Autodesk Inventor part; units mm, degrees
ref_plane "YZ Plane" through (0, 0, 0) normal (1, 0, 0) x (0, 1, 0)
ref_plane "XZ Plane" through (0, 0, 0) normal (0, 1, 0) x (-1, 0, 0)
ref_plane "XY Plane" through (0, 0, 0) normal (0, 0, 1) x (1, 0, 0)
sketch "Sketch1" plane through (0, 0, 0) normal (0, 0, 1) x (1, 0, 0)
  line L0 (0, 0) -> (18, 0)
  line L1 (18, 0) -> (18, 24)
  line L2 (18, 24) -> (0, 24)
  line L3 (0, 24) -> (0, 0)
  circle A0 centre (15, 21) radius 1.05
  circle A1 centre (5, 2.5) radius 1.05
  circle A2 centre (3, 7) radius 1.05
  line L4 (0, 10) -> (11.3137, 10) construction
  line L5 (6, 0) -> (28.3492, 0) construction
  line L6 (6, 0) -> (42, 0) construction
  circle A3 centre (9.749, 12) radius 1
  circle A4 centre (15, 21) radius 2.75
  circle A5 centre (5, 5) radius 5
  line L7 (1.1063, 8.1367) -> (12.8585, 22.7252)
  circle A6 centre (5, 2.5) radius 2.5
  line L8 (7.185, 1.2851) -> (17.4035, 19.6637)
  point P0 (8, 24)
  point P1 (18, 31.1769)
  point P2 (9.5257, 2.8745)
  point P3 (17.4892, 19.831)
  point P4 (5, 0)
  dimension "d0" = 18
  dimension "d1" = 24
  dimension "d2" = 2.1
  dimension "d3" = 3
  dimension "d4" = 3
  dimension "d5" = 2.1
  dimension "d6" = 2.1
  dimension "d7" = 2.5
  dimension "d8" = 5
  dimension "d9" = 3
  dimension "d10" = 7
  dimension "d12" = 10
  dimension "d15" = 6
  dimension "d18" = 2
  dimension "d25" = 5.5
  dimension "d26" = 10
  dimension "d30" = 12
  dimension "d31" = 8.251
extrude "Extrusion1" add sketch "Sketch1" along normal blind 8 contours A5 L8 A6 | A6 | L7 A4 L8 A5 | A4 picked at (5.8937, 6.9979)
sketch "Sketch3" plane through (0, 0, 0) normal (0, 0, -1) x (-1, 0, 0)
  circle A0 centre (-9.749, 12) radius 1
  circle A1 centre (-9.749, 12) radius 7.45
  point P0 (0, 0)
  dimension "d27" = 14.9
extrude "Extrusion2" cut sketch "Sketch3" against normal blind 2.7
sketch "Sketch5" plane through (0, 0, 8) normal (0, 0, 1) x (1, 0, 0)
  circle A0 centre (3, 7) radius 1.05
  circle A1 centre (5, 2.5) radius 1.05
  circle A2 centre (15, 21) radius 1.05
  circle A3 centre (3, 7) radius 2
  circle A4 centre (5, 2.5) radius 2
  circle A5 centre (15, 21) radius 2
  point P0 (0, 0)
  dimension "d32" = 4
  dimension "d33" = 4
  dimension "d34" = 4
extrude "Extrusion3" cut sketch "Sketch5" against normal blind 4.9
sketch "Sketch6" plane through (0, 0, 2.7) normal (0, 0, -1) x (-1, 0, 0)
  circle A0 centre (-9.749, 12) radius 1
  circle A1 centre (-9.749, 12) radius 1
  circle A2 centre (-9.749, 12) radius 5.7
  point P0 (0, 0)
  dimension "d37" = 11.4
extrude "Extrusion4" cut sketch "Sketch6" against normal blind 3.65
sketch "Sketch8" plane through (1.1063, 8.1367, 0) normal (-0.778745, 0.6273406, 0) x (0, 0, 1)
  line L0 (0, 21.4833) -> (8, 21.4833)
  line L1 (8, 18.7333) -> (8, 0)
  line L2 (8, 18.7333) -> (8, 21.4833)
  line L3 (4, 21.4833) -> (8, 15)
  line L4 (8, -1.5222) -> (8, 19.2005)
  point P0 (0, -7.0304)
  point P1 (8, 15)
extrude "Extrusion5" cut sketch "Sketch8" against normal up to surface surface through (7.185, 1.2851, 0) normal (0.8739914, -0.4859413, 0)
properties part number "PartD_3D"
Geometry check sheet. Reference: the model listing, model coordinates, mm. A direction names the side the tool comes from. Round coordinates to 2 decimals unless told otherwise and drop trailing zeros. Loops run counter-clockwise (first coordinate to the right, second up) from the corner with the lowest first, then second, coordinate; pieces in that order, holes last. Notation, with made-up numbers: (-34, -30) -> (-6, -30) arc R21 cw to (-6, -18) -> close; hole circle Ø8 at (1.5, 5.25). An arc over 180 degrees is marked (long way). Answer as a JSON object with one key per item and string values. Group by question number.
Item 1: Depth check by flat-ended pin: pin 1 Ø3 at (y, z) = (17, 5) entering from -X; pin 2 Ø2.5 at (x, y) = (5, 2.5) entering from -Z; pin 3 Ø1.5 at (y, z) = (17, 1.5) entering from -X; pin 4 Ø2 at (x, y) = (7, 6.5) entering from -Z. Enter the tip coordinate at first touch or a pass-through.
Item 2: Cross-section at A-A, the plane z = 0.5. Count the separate pieces of the cut face and the enclosed holes in it, plus the area to 3 significant figures.
Item 3: Set-up check for faces 1 (the face through (6, 7, 2.7)), 2 (the face through (13.211, 18.597, 1.331)), 3 (the face through (12.123, 17.182, 4.499)), 4 (the face through (13.4, 19.8, 4.6)): record each of +Z, -Z, +X, -X, +Y, -Y from which the full face is reachable in a straight line by a thin tool's end or side.
Item 4: Cross-section at C-C, the plane y = 2.25. Record the cut outline in (x, z), plus the area to 3 significant figures.
Item 5: Release check for a two-part mould opening along Y. For faces 5 (the face through (8, 12, 6.35)), 6 (the face through (14, 20, 0)), 7 (the face through (2.98, 8.89, 1.33)) record: pulls with the +Y half, pulls with the -Y half, needs draft (parallel to the pull), parting line crosses it, or undercut.
Item 6: Cross-section at B-B, the plane x = 15. Record the cut outline in (y, z).
Item 7: Thickness scan on line 1 along Y through (x, z) = (4.5, 5.5); line 2 along Z through (x, y) = (16.5, 19.75); line 3 along X through (y, z) = (21.5, 3.75). Record the ranges inside material, lowest first.
Item 8: Cross-section at D-D, the plane x = 7.5. Record the cut outline in (y, z), plus the area to 3 significant figures.
Determined:
{
 "1": {"pin 1": "stops at x = 7.72", "pin 2": "stops at z = 0", "pin 3": "stops at x = 14.49", "pin 4": "stops at z = 2.7"},
 "2": {"separate pieces": "2", "enclosed holes": "2", "area": "69.2 mm²"},
 "3": {"face 1": "-Z, +X, +Y", "face 2": "-Z, -X, -Y", "face 3": "-Z", "face 4": "+Z"},
 "4": {"outline": "(0.82, 0) -> (3.98, 0) -> (3.98, 3.1) -> (3.02, 3.1) -> (3.02, 8) -> (0.82, 8) -> close; (6.02, 0) -> (7.72, 0) -> (7.72, 8) -> (6.98, 8) -> (6.98, 3.1) -> (6.02, 3.1) -> close", "area": "29.4 mm²"},
 "5": {"face 5": "undercut", "face 6": "needs draft", "face 7": "pulls with the +Y half"},
 "6": {"outline": "(15.34, 2.7) -> (17.28, 2.7) -> (17.28, 0) -> (19.95, 0) -> (19.95, 3.1) -> (19, 3.1) -> (19, 6.66) -> (16.21, 8) -> (15.34, 8) -> close; (22.05, 0) -> (23.75, 0) -> (23.75, 4.38) -> (23, 4.74) -> (23, 3.1) -> (22.05, 3.1) -> close"},
 "7": {"line 1": "y = 0.03 to 0.56, 4.44 to 5.68, 8.32 to 9.78", "line 2": "z = 0 to 3.1", "line 3": "x = 11.87 to 13.06, 16.94 to 17.7"},
 "8": {"outline": "(1.85, 0) -> (4.9, 0) -> (4.9, 2.7) -> (6.76, 2.7) -> (6.76, 6.35) -> (16.07, 6.35) -> (16.07, 8) -> (1.85, 8) -> close", "area": "49.6 mm²"}
}
